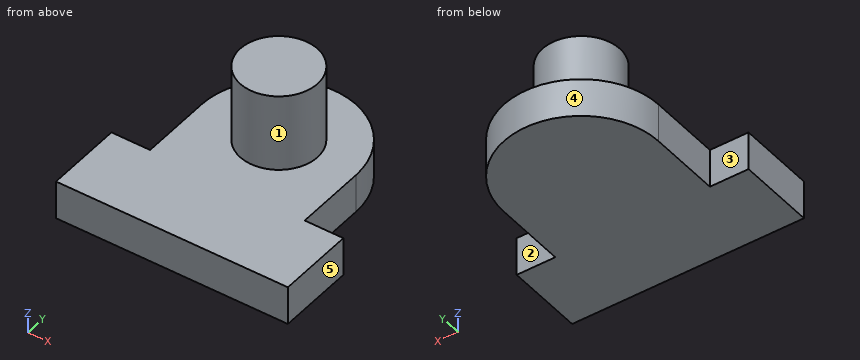
from build123d import *

# Parameters (mm, degrees)
BOSS_EXTRUDE1_DEPTH = 10
SKETCH3_R           = 10
BOSS_EXTRUDE2_DEPTH = 20


with BuildPart() as part:
    # Sketch2 → Boss-Extrude1 (new body)
    with BuildSketch(Plane.XY):
        with BuildLine():
            Line((0, 0), (10, 0))
            Line((10, 0), (10, 18.56))
            ThreePointArc((10, 18.56), (30, 38.56), (50, 18.56))
            Line((50, 18.56), (50, 0))
            Line((50, 0), (60, 0))
            Line((60, 0), (60, -20))
            Line((60, -20), (0, -20))
            Line((0, -20), (0, 0))
        make_face()
    extrude(amount=BOSS_EXTRUDE1_DEPTH)

    # Sketch3 → Boss-Extrude2 (add)
    with BuildSketch(Plane.XY.offset(10)):
        with Locations(Location((30, 18.56, 0), (0, 0, 180))):
            Circle(SKETCH3_R)
    extrude(amount=BOSS_EXTRUDE2_DEPTH)


solid = part.part
Work out the finished part from the listing and answer in its coordinate system (mm). Face numbers are marked on the shaded views. A direction names the side the tool comes from. Give positions to 0.01 mm unless a question says otherwise; leave off trailing zeros. Loops run counter-clockwise (first coordinate to the right, second up) from the corner with the lowest first, then second, coordinate; pieces in that order, holes last. Notation, with made-up numbers: M -19,75.5 L 34,75.5 A9 ccw 34,90.5 Z; hole C 80,59.25 d9. An arc over 180 degrees is marked long. Use CSV: the item, a comma, the result in double quotes.
1) Find section B-B on z = 26.5. Write down the section's boundary in (x, y).
Answer:
outline,"C 30,18.56 d20"
2) Find section D-D on x = 14. Write down the section's boundary in (y, z), plus the area to 3 significant figures.
Answer:
outline,"M -20,0 L 30.56,0 L 30.56,10 L -20,10 Z"
area,"506 mm^2"
3) Consider L1, parallel to Z at x = 21, y = -15; L2, parallel to Y at x = 54, z = 5.25; L3, parallel to X at y = 6, z = 4.75. Determine where each line is inside the solid, lowest interval first.
Answer:
L1,"0 to 10"
L2,"-20 to 0"
L3,"10 to 50"
4) Find section C-C on y = 20. Write down the section's boundary in (x, z), plus the area to 3 significant figures.
Answer:
outline,"M 10.05,0 L 49.95,0 L 49.95,10 L 39.9,10 L 39.9,30 L 20.1,30 L 20.1,10 L 10.05,10 Z"
area,"795 mm^2"
5) Which of the six approach directions +Z, -Z, +X, -X, +Y, -Y give full straight-line access (tool end or side, diameter ignored) to the marked faces 1, 2, 3, 4 and 5?
Answer:
face 1,"+Z"
face 2,"+Z, -Z, +X, +Y"
face 3,"+Z, -Z, -X, +Y"
face 4,"+Z, -Z, +Y"
face 5,"+Z, -Z, +X, +Y, -Y"
6) Given P1, Ø12, axis at x = 29, z = 9.5, coming from the +Y side; P2, Ø3, axis at x = 53.5, z = 2.5, coming from the +Y side; P3, Ø5, axis at y = 6, z = 5, coming from the +X side; P4, Ø4, axis at y = 32, z = 23.5, coming from the +X side, each flat-ended and moving along its own axis, determine where each tip first touches the part or whether it passes through.
Answer:
P1,"y = 38.56"
P2,"y = 0"
P3,"x = 50"
P4,"through"
7) Find section A-A on x = 30. Write down the section's boundary in (y, z), plus the area to 3 significant figures.
Answer:
outline,"M -20,0 L 38.56,0 L 38.56,10 L 28.56,10 L 28.56,30 L 8.56,30 L 8.56,10 L -20,10 Z"
area,"986 mm^2"
